Can you work these out from the model? Positions are in its coordinate system, mm. Round coordinates to 2 decimals unless told otherwise and drop trailing zeros. Loops run counter-clockwise (first coordinate to the right, second up) from the corner with the lowest first, then second, coordinate; pieces in that order, holes last.
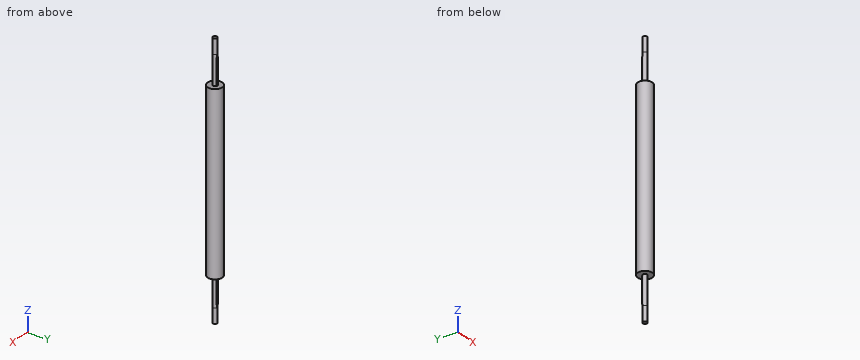
from build123d import *
from build123d.topology import SkipClean

# Parameters (mm, degrees)
BOSS_EXTRUDE4_DEPTH = 800
SKETCH6_R           = 50
BOSS_EXTRUDE5_DEPTH = 600
BOSS_EXTRUDE6_START = 900
SKETCH7_R           = 15
BOSS_EXTRUDE6_DEPTH = 100
CUT_EXTRUDE1_DEPTH  = 20
CUT_EXTRUDE2_START  = -20
CUT_EXTRUDE2_DEPTH  = 20


with BuildPart() as part:
    # Sketch4 → Boss-Extrude4 (new, symmetric)
    with BuildSketch(Plane.XY):
        with BuildLine():
            Line((-5, 14.142135624), (-5, 18.3))
            Line((-5, 18.3), (5, 18.3))
            Line((5, 18.3), (5, 14.142135624))
            ThreePointArc((5, 14.142135624), (0, -15), (-5, 14.142135624))
        make_face()
    extrude(amount=BOSS_EXTRUDE4_DEPTH, both=True)

    # Sketch6 → Boss-Extrude5 (add, symmetric)
    with BuildSketch(Plane.XY):
        Circle(SKETCH6_R)
    extrude(amount=BOSS_EXTRUDE5_DEPTH, both=True)

    # Sketch7 → Boss-Extrude6 (add)
    with BuildSketch(Plane.XY.offset(BOSS_EXTRUDE6_START)):
        with Locations(Location((0, 0, 0), (0, 0, 109.471220634))):
            Circle(SKETCH7_R)
    boss_extrude6 = extrude(amount=-BOSS_EXTRUDE6_DEPTH)

    # Mirror1: Boss-Extrude6 across plane
    add(boss_extrude6.mirror(Plane.XY))

    # Sketch8 → Cut-Extrude1 (cut)
    with BuildSketch(Plane.XY.offset(800)):
        with BuildLine():
            Line((5, 14.142135624), (5, 18.3))
            Line((5, 18.3), (-5, 18.3))
            Line((-5, 18.3), (-5, 14.142135624))
            ThreePointArc((-5, 14.142135624), (0, 15), (5, 14.142135624))
        make_face()
    extrude(amount=-CUT_EXTRUDE1_DEPTH, mode=Mode.SUBTRACT)

    # Sketch9 → Cut-Extrude2 (cut)
    with SkipClean():  # the faces are left unmerged after this step: merging them gives an invalid solid
        with BuildSketch(Plane(origin=(0, 0, -800), x_dir=(-1, 0, 0), z_dir=(0, 0, -1)).offset(CUT_EXTRUDE2_START)):
            with BuildLine():
                Line((-5, 18.3), (-5, 14.142135624))
                ThreePointArc((-5, 14.142135624), (0, 15), (5, 14.142135624))
                Line((5, 14.142135624), (5, 18.3))
                Line((5, 18.3), (-5, 18.3))
            make_face()
        extrude(amount=CUT_EXTRUDE2_DEPTH, mode=Mode.SUBTRACT)


solid = part.part
(1) If we section it at A-A, the plane z = -683: List the corners of the cut face in (x, y) for me.
Worked answers:
outline: (-5, 14.14) arc R15 ccw (long way) to (5, 14.14) - (5, 18.3) - (-5, 18.3) - close
(2) If I drill on line 1 (Z direction, x = 29, y = 15.5); line 2 (Y direction, x = -5, z = -356.5); line 3 (X direction, y = -16, z = 527.5), over which ranges is the centre line in solid material (lowest first)?
Worked answers:
line 1: z = -600 to 600
line 2: y = -49.75 to 49.75
line 3: x = -47.37 to 47.37
(3) Will these pins go through, and if not, where does the flat tip stop? P1, Ø3.5, axis at y = 17, z = 710.5, coming from the -X side; P2, Ø1, axis at y = 31, z = 376.5, coming from the -X side; P3, Ø3.5, axis at y = 15.5, z = -656.5, coming from the -X side.
Worked answers:
P1: stops at x = -5
P2: stops at x = -39.62
P3: stops at x = -5.99
(4) If we section it at B-B, the plane z = -55: List the corners of the cut face in (x, y) for me.
Worked answers:
outline: circle Ø100 at (0, 0)
